from build123d import *

# Parameters (mm, degrees)
SKETCH1_W          = 25.4
SKETCH1_H          = 22.225
EXTRUDE1_DEPTH     = 1.5875
SKETCH2_R          = 3.571875
CUT_EXTRUDE1_DEPTH = 4.175


with BuildPart() as part:
    # Sketch1 → Extrude1 (new body, symmetric)
    with BuildSketch(Plane(origin=(0, 0, 0), x_dir=(1, 0, 0), z_dir=(0, 1, 0))):
        Rectangle(SKETCH1_W, SKETCH1_H)
    extrude(amount=EXTRUDE1_DEPTH, both=True)

    # Sketch2 → Cut-Extrude1 (cut, through all)
    with BuildSketch(Plane(origin=(0, 1.5875, 0), x_dir=(1, 0, 0), z_dir=(0, 1, 0))):
        Circle(SKETCH2_R)
    extrude(amount=-CUT_EXTRUDE1_DEPTH, mode=Mode.SUBTRACT)


solid = part.part
Work out the finished part from the listing and answer in its coordinate system (mm). Round coordinates to 2 decimals unless told otherwise and drop trailing zeros. Write each loop counter-clockwise with the first axis right and the second up, starting at its lowest first coordinate (ties: lowest second). Pieces come first, ordered by that corner, then holes. Notation, with made-up numbers: (50.5, 60.25) - (104.5, 60.25) arc R30 ccw to (104.5, 96.25) - close; hole circle Ø3 at (64.5, 19.25). An arc over 180 degrees is marked (long way). Answer in a Markdown table with one row per item. Add a question column.
1. A cutting plane is placed at B-B, the plane x = 0. Determine the outline of the cut face in (y, z).
2. Find the intervals of material crossed by line 1 along X through (y, z) = (-0.2, 0); line 2 along Z through (x, y) = (0, -0.9); line 3 along Z through (x, y) = (-1.25, 0), in increasing order. Write a range as from..to.
3. A cutting plane is placed at A-A, the plane z = 0. Determine the outline of the cut face in (x, y), and give its area (3 significant figures).
4. The mould has two halves that part along X. Classify faces 1 (the cylindrical face through (-3.57, 0.02, -0.16)), 2 (the flat face through (-12.7, 0, 0)), 3 (the flat face through (-3, -1.588, -3)): +X half, -X half, draft (parallel to the pull), parting line (faces both ways), or undercut.
5. Given pin 1 (4.5 mm diameter, centred on x = 0, z = 0, fed in from -Y), flat-ended and moving along its own axis, determine where the tip first touches the part or whether it passes through.
6. A cutting plane is placed at C-C, the plane y = -1.1. Determine the outline of the cut face in (x, z), and give its area (3 significant figures).
Worked out:
| question | item | result |
|---|---|---|
| 1 | outline | (-1.59, -11.11) - (1.59, -11.11) - (1.59, -3.57) - (-1.59, -3.57) - close; (-1.59, 3.57) - (1.59, 3.57) - (1.59, 11.11) - (-1.59, 11.11) - close |
| 2 | line 1 | -12.7..-3.57, 3.57..12.7 |
| 2 | line 2 | -11.11..-3.57, 3.57..11.11 |
| 2 | line 3 | -11.11..-3.35, 3.35..11.11 |
| 3 | outline | (-12.7, -1.59) - (-3.57, -1.59) - (-3.57, 1.59) - (-12.7, 1.59) - close; (3.57, -1.59) - (12.7, -1.59) - (12.7, 1.59) - (3.57, 1.59) - close |
| 3 | area | 58.0 mm^2 |
| 4 | face 1 | undercut |
| 4 | face 2 | -X half |
| 4 | face 3 | draft |
| 5 | pin 1 | through |
| 6 | outline | (-12.7, -11.11) - (12.7, -11.11) - (12.7, 11.11) - (-12.7, 11.11) - close; hole circle Ø7.14 at (0, 0) |
| 6 | area | 524 mm^2 |
